```python
from build123d import *

# Parameters (mm, degrees)
F0_W      = 135
F0_H      = 90
F1_DEPTH  = 3
F3_R      = 1.75
F4_DEPTH  = 3.001
F5_R      = 1.575
F6_DEPTH  = 3
F7_W      = 38.05
F7_H      = 15
F8_DEPTH  = 3
F9_R      = 1.375
F10_DEPTH = 3
F11_W     = 31.8
F11_H     = 40
F12_DEPTH = 3
F13_W     = 15
F13_H     = 50
F13_R     = 1.5
F14_DEPTH = 3
F15_R     = 3
F16_R     = 0.49999
F17_R     = 5
F18_R     = 1.875
F19_DEPTH = 3.001


# Not quite as in the source:
# - a fillet or chamfer is up to 0.001 mm smaller than in the source, because OpenCascade refuses the exact size
# - a feature names something its author has since deleted; it is built from what else it names


with BuildPart() as f1:
    # F0 (on Top) → F1 (new body)
    with BuildSketch(Plane.XY):
        Rectangle(F0_W, F0_H)
    extrude(amount=F1_DEPTH)

    # F3 (on face) → F4 (cut, through all)
    with BuildSketch(Plane.XY.offset(3)):
        with Locations((-59.5, 11)):
            Circle(F3_R)
        with Locations((19.5, 11)):
            Circle(F3_R)
        with Locations((19.5, -31)):
            Circle(F3_R)
        with Locations((-59.5, -31)):
            Circle(F3_R)
    extrude(amount=-F4_DEPTH, mode=Mode.SUBTRACT)

    # F5 (on Top) → F6 (join, through all)
    with BuildSketch(Plane.XY):
        Polygon((-37.8, 46), (-37.8, 45), (37.8, 45), (37.8, 46), (61.2, 46), (61.2, 60), (37.8, 60), (-37.7553022623, 60), (-37.8, 60), (-61.2, 60), (-61.2, 46), align=None)
        with Locations((-55, 52.5)):
            Circle(F5_R, mode=Mode.SUBTRACT)
        with Locations((-35.6, 52.5)):
            Circle(F5_R, mode=Mode.SUBTRACT)
        with Locations((35.6, 52.5)):
            Circle(F5_R, mode=Mode.SUBTRACT)
        with Locations((55, 52.5)):
            Circle(F5_R, mode=Mode.SUBTRACT)
        Polygon((37.8, -46), (37.8, -45), (-37.8, -45), (-37.8, -46), (-61.2, -46), (-61.2, -60), (-37.8, -60), (-37.7553022623, -60), (37.8, -60), (61.2, -60), (61.2, -46), align=None)
        with Locations((-55, -52.5)):
            Circle(F5_R, mode=Mode.SUBTRACT)
        with Locations((-35.6, -52.5)):
            Circle(F5_R, mode=Mode.SUBTRACT)
        with Locations((35.6, -52.5)):
            Circle(F5_R, mode=Mode.SUBTRACT)
        with Locations((55, -52.5)):
            Circle(F5_R, mode=Mode.SUBTRACT)
    extrude(amount=F6_DEPTH)

    # F7 (on face) → F8 (cut, through all)
    with BuildSketch(Plane.XY.offset(3)):
        with Locations((0, -52.5)):
            Rectangle(F7_W, F7_H)
        with Locations((0, 52.5)):
            Rectangle(F7_W, F7_H)
    extrude(amount=-F8_DEPTH, mode=Mode.SUBTRACT)

    # F9 (on face) → F10 (cut, through all)
    with BuildSketch(Plane.XY.offset(3)):
        with Locations((-61.4022165537, 41.125)):
            Circle(F9_R)
        with Locations((-54.9034181798, 41.2499787819)):
            Circle(F9_R)
        with Locations((-24.2189181921, -35.6262016261)):
            Circle(F9_R)
        with Locations((-24.0939394102, -42.125)):
            Circle(F9_R)
        with Locations((-12.5939394102, -42.125)):
            Circle(F9_R)
        with Locations((-12.7189181921, -35.6262016261)):
            Circle(F9_R)
        with Locations((-1.0939394102, -42.125)):
            Circle(F9_R)
        with Locations((-1.2189181921, -35.6262016261)):
            Circle(F9_R)
        with Locations((10.4060605898, -42.125)):
            Circle(F9_R)
        with Locations((10.2810818079, -35.6262016261)):
            Circle(F9_R)
        with Locations((21.9060605898, -42.125)):
            Circle(F9_R)
        with Locations((21.7810818079, -35.6262016261)):
            Circle(F9_R)
    extrude(amount=-F10_DEPTH, mode=Mode.SUBTRACT)

    # F11 (on face) → F12 (cut, through all)
    with BuildSketch(Plane.XY.offset(3)):
        with Locations((-20.9, -4.4738012552)):
            Rectangle(F11_W, F11_H)
    extrude(amount=-F12_DEPTH, mode=Mode.SUBTRACT)

    # F13 (on Top) → F14 (join, through all)
    with BuildSketch(Plane.XY):
        with Locations((75, 0)):
            Rectangle(F13_W, F13_H)
        with Locations((70, -12.5)):
            Circle(F13_R, mode=Mode.SUBTRACT)
        with Locations((80, -12.5)):
            Circle(F13_R, mode=Mode.SUBTRACT)
        with Locations((70, 12.5)):
            Circle(F13_R, mode=Mode.SUBTRACT)
        with Locations((80, 12.5)):
            Circle(F13_R, mode=Mode.SUBTRACT)
    extrude(amount=F14_DEPTH)

    # F15
    f15_edges = [f1.edges().sort_by_distance(p)[0] for p in [
        (-36.8, -24.473801, 1.5),
        (-5, -24.473801, 1.5),
        (-5, 15.526199, 1.5),
        (-36.8, 15.526199, 1.5),
    ]]
    fillet(f15_edges, radius=F15_R)

    # F16 (radius 0.5 in the source; OpenCascade refuses exactly that, so slightly less here)
    f16_edges = [f1.edges().sort_by_distance(p)[0] for p in [
        (-37.8, 46, 1.5),
        (-37.8, 45, 1.5),
        (37.8, 46, 1.5),
        (37.8, 45, 1.5),
        (37.8, -45, 1.5),
        (37.8, -46, 1.5),
        (-37.8, -46, 1.5),
        (-37.8, -45, 1.5),
    ]]
    fillet(f16_edges, radius=F16_R)

    # F17
    f17_edges = [f1.edges().sort_by_distance(p)[0] for p in [
        (-19.025, -60, 1.5),
        (-19.025, -45, 1.5),
        (-61.2, -60, 1.5),
        (-61.2, -46, 1.5),
        (-67.5, -45, 1.5),
        (19.025, -60, 1.5),
        (19.025, -45, 1.5),
        (61.2, -60, 1.5),
        (61.2, -46, 1.5),
        (67.5, -45, 1.5),
        (61.2, 46, 1.5),
        (67.5, 45, 1.5),
        (61.2, 60, 1.5),
        (19.025, 45, 1.5),
        (19.025, 60, 1.5),
        (-19.025, 45, 1.5),
        (-19.025, 60, 1.5),
        (-61.2, 46, 1.5),
        (-61.2, 60, 1.5),
        (-67.5, 45, 1.5),
        (67.5, -25, 1.5),
        (82.5, -25, 1.5),
        (67.5, 25, 1.5),
        (82.5, 25, 1.5),
    ]]
    fillet(f17_edges, radius=F17_R)

    # F18 (on face) → F19 (cut, through all)
    with BuildSketch(Plane.XY.offset(3)):
        with Locations((-34.975, 35)):
            Circle(F18_R)
        with Locations((34.975, 35)):
            Circle(F18_R)
    extrude(amount=-F19_DEPTH, mode=Mode.SUBTRACT)


solid = f1.part
```
The model under review builds one solid part; all positions refer to its coordinate system, in mm. A direction names the side the tool comes from. Round coordinates to 2 decimals unless told otherwise and drop trailing zeros. Loops run counter-clockwise (first coordinate to the right, second up) from the corner with the lowest first, then second, coordinate; pieces in that order, holes last.
1) Consider section B-B on y = 7. State the section outline as (x, z) points, then the cut area to 3 significant figures.
Values follow:
outline: (-67.5, 0) - (-36.8, 0) - (-36.8, 3) - (-67.5, 3) - close; (-5, 0) - (82.5, 0) - (82.5, 3) - (-5, 3) - close
area: 355 mm2
2) Wall thickness on line 1 along Y through (x, z) = (55, 2) (3 decimals); line 2 along Y through (x, z) = (39, 1.85); line 3 along Y through (x, z) = (-17, 1.05): over which ranges is each line inside the solid? List them lowest first.
Values follow:
line 1: y = -60 to -54.075, -50.925 to -46, -45 to 45, 46 to 50.925, 54.075 to 60
line 2: y = -60 to -46, -45 to 45, 46 to 60
line 3: y = -45.98 to -24.47, 15.53 to 45.98
3) Consider section A-A on y = 35. State the section outline as (x, z) points.
Values follow:
outline: (-67.5, 0) - (-36.85, 0) - (-36.85, 3) - (-67.5, 3) - close; (-33.1, 0) - (33.1, 0) - (33.1, 3) - (-33.1, 3) - close; (36.85, 0) - (67.5, 0) - (67.5, 3) - (36.85, 3) - close
4) The part is to be moulded in two halves that separate along Y. For faces 5 (the face through (67.5, -35, 1)), 6 (the face through (-21, -24.474, 2)), 7 (the face through (-20.529, 58.574, 1.479)), say which applies: pulls with the +Y half, pulls with the -Y half, needs draft (parallel to the pull), parting line crosses it, or undercut.
Values follow:
face 5: needs draft
face 6: undercut
face 7: pulls with the +Y half
5) Clearance check with flat-ended pins moving along their axes: P1, Ø3, axis at x = -59.5, y = -31, coming from the +Z side; P2, Ø1, axis at y = -33.5, z = 2, coming from the +X side; P3, Ø0.9, axis at x = 74, z = 2, coming from the -Y side; P4, Ø0.9, axis at y = 52.5, z = 1.5, coming from the +X side. State where each tip first meets the part, or that it passes through.
Values follow:
P1: passes through
P2: stops at x = 67.5
P3: stops at y = -25
P4: stops at x = 61.2
6) Consider section D-D on x = 6. State the section outline as (y, z) points, then the cut area to 3 significant figures.
Values follow:
outline: (-45, 0) - (45, 0) - (45, 3) - (-45, 3) - close
area: 270 mm2
7) Consider section C-C on z = 1.2. Give the number of separate pieces and of enclosed holes in the cut face, then the cut area to 3 significant figures.
Values follow:
separate pieces: 1
enclosed holes: 31
area: 13,800 mm2
8) Tool access review of faces 1 (the face through (61.2, 53, 1)), 2 (the face through (20.451, -58.496, 1.479)), 3 (the face through (0, 45, 2)), 4 (the face through (-61.2, 53, 1)): name each direction out of +Z, -Z, +X, -X, +Y, -Y from which nothing blocks a thin tool from reaching the whole face with its end or side.
Values follow:
face 1: +Z, -Z, +X, +Y
face 2: +Z, -Z, -Y
face 3: +Z, -Z, +Y
face 4: +Z, -Z, -X, +Y
